CAD build for the part. Positions are in the model's coordinates, mm. A direction names the side the tool comes from. Give positions to 0.01 mm unless a question says otherwise; leave off trailing zeros. Loops run counter-clockwise (first coordinate to the right, second up) from the corner with the lowest first, then second, coordinate; pieces in that order, holes last. Notation, with made-up numbers: M -3,75.5 L 21,75.5 A34 cw 21,106.5 Z; hole C -39.75,62.25 d11. An arc over 180 degrees is marked long. Answer as CSV lines item,"result".
from build123d import *

# Parameters (mm, degrees)
SKETCH3_R          = 1.5
CUT_EXTRUDE1_DEPTH = 10
CIRPATTERN1_COUNT  = 3


with BuildPart() as part:
    # Sketch2 → Revolve1 (revolve)
    with BuildSketch(Plane.XY, mode=Mode.PRIVATE) as revolve1_sk:
        Polygon((14, 15), (11, 15), (11, 5), (0, 5), (0, 0.75), (14, 0.75), align=None)
    revolve(revolve1_sk.sketch.rotate(Axis((0, 0, 0), (1, 0, 0)), 90), axis=Axis((0, 0, 0), (1, 0, 0)))

    # Sketch3 → Cut-Extrude1 (cut)
    with BuildSketch(Plane.ZY.offset(-11)):
        with Locations((0, 10)):
            Circle(SKETCH3_R)
    cut_extrude1 = extrude(amount=-CUT_EXTRUDE1_DEPTH, mode=Mode.SUBTRACT)

    # CirPattern1: Cut-Extrude1 ×3 about axis
    cirpattern1_axis = Axis((0, 0, 0), (1, 0, 0))
    for i in range(1, CIRPATTERN1_COUNT):
        add(cut_extrude1.rotate(cirpattern1_axis, i * 360 / CIRPATTERN1_COUNT), mode=Mode.SUBTRACT)


solid = part.part
1) Drill centre lines: line 1 (Y direction, x = 12.05, z = 0); line 2 (Y direction, x = 12, z = 0.5); line 3 (X direction, y = -9, z = -6.5). Where is each one in solid material? Low to high. Write a range as from..to.
Answer below:
line 1,"y = -15..-0.75, 0.75..8.5, 11.5..15"
line 2,"y = -14.99..-0.56, 0.56..8.59, 11.41..14.99"
line 3,"x = 11..14"
2) Flat gauge pins, fed straight in: pin 1 (4 mm diameter, centred on x = 1.5, z = 2.5, fed in from +Y); pin 2 (1.8 mm diameter, centred on y = 10, z = 0, fed in from -X); pin 3 (1 mm diameter, centred on y = 6, z = -8.5, fed in from -X); pin 4 (1.5 mm diameter, centred on x = 11.5, z = -4.5, fed in from +Y). Where does each tip first touch, or does it go through?
Answer below:
pin 1,"stops at y = 4.97"
pin 2,"passes through"
pin 3,"stops at x = 11"
pin 4,"stops at y = 14.52"
3) Band-saw the part on A-A on z = 0. Give the cut face in (x, y).
Answer below:
outline,"M 0,-5 L 11,-5 L 11,-15 L 14,-15 L 14,-0.75 L 0,-0.75 Z; M 0,0.75 L 14,0.75 L 14,8.5 L 11,8.5 L 11,5 L 0,5 Z; M 11,11.5 L 14,11.5 L 14,15 L 11,15 Z"
4) Band-saw the part on C-C on x = 7.25. Give the cut face in (y, z), and give its area (3 significant figures).
Answer below:
outline,"C 0,0 d10; hole C 0,0 d1.5"
area,"76.8 mm^2"
5) Mould opens along Z. For faces 1 (the face through (14, 0, -3)), 2 (the face through (7.098, -0.225, 0.715)), 3 (the face through (12.48, -5.91, 7.47)), 4 (the face through (12.48, -12.65, 8.06)) say: +Z half, -Z half, draft (parallel to the pull), parting line (faces both ways), or undercut.
Answer below:
face 1,"draft"
face 2,"undercut"
face 3,"undercut"
face 4,"parting line"
6) Which spindle directions (+Z, -Z, +X, -X, +Y, -Y) get a long thin tool onto all of the face, cutting with end or side? Do faces 5 (the face through (11, -4, -4)), 6 (the face through (0, 0, 1)). Say none if no direction does.
Answer below:
face 5,"-X"
face 6,"+Z, -Z, -X, +Y, -Y"
7) Band-saw the part on D-D on x = 13.25. Give the cut face in (y, z), and give its area (3 significant figures).
Answer below:
outline,"C 0,0 d30; hole C -5,-8.66 d3; hole C -5,8.66 d3; hole C 0,0 d1.5; hole C 10,0 d3"
area,"684 mm^2"
8) Band-saw the part on B-B on y = 0. Give the cut face in (x, z), and give its area (3 significant figures).
Answer below:
outline,"M 0,-5 L 11,-5 L 11,-15 L 14,-15 L 14,-0.75 L 0,-0.75 Z; M 0,0.75 L 14,0.75 L 14,15 L 11,15 L 11,5 L 0,5 Z"
area,"179 mm^2"
